Geometry: final body of the model. Coordinates: model frame, mm. A direction names the side the tool comes from. Give positions to 0.01 mm unless a question says otherwise; leave off trailing zeros. Write each loop counter-clockwise with the first axis right and the second up, starting at its lowest first coordinate (ties: lowest second). Pieces come first, ordered by that corner, then holes. Notation, with made-up numbers: (1, 64) - (21, 64) arc R26 cw to (21, 101) - close; hole circle Ø4 at (5.5, 23.5). An arc over 180 degrees is marked (long way). Return JSON: item names as keys, results as strings.
from build123d import *

# Parameters (mm, degrees)
BOSS_EXTRUDE5_DEPTH = 234.9999999
SKETCH4_W           = 42.5
SKETCH4_H           = 48.09999997
CUT_EXTRUDE1_DEPTH  = 2.000000064


with BuildPart() as part:
    # Sketch1 → Boss-Extrude5 (new body)
    with BuildSketch(Plane(origin=(0, 0, 0), x_dir=(1, 0, 0), z_dir=(0, 1, 0))):
        Polygon((-117.504462868, 326.155640462), (117.504462868, 326.155640462), (263.000000064, 160.754471715), (263.000000064, 45.003453118), (261, 45.003453118), (261, 160), (116.600094822, 324.155640398), (-116.600094822, 324.155640398), (-261, 160), (-261, 45.001214275), (-263.000000064, 45.001214275), (-263.000000064, 160.754471715), align=None)
    extrude(amount=BOSS_EXTRUDE5_DEPTH)

    # Sketch4 → Cut-Extrude1 (cut)
    with BuildSketch(Plane(origin=(0, 0, -326.155640462), x_dir=(-1, 0, 0), z_dir=(0, 0, -1))):
        with Locations((0, 87.449999931)):
            Rectangle(SKETCH4_W, SKETCH4_H)
        Polygon((-25, 63.399999946), (-25, 28.4), (25, 28.4), (25, 63.399999946), (21.25, 63.399999946), (-21.25, 63.399999946), align=None)
        Polygon((-25, 28.4), (-35, 28.4), (-35, 0), (35, 0), (35, 28.4), (25, 28.4), align=None)
    extrude(amount=-CUT_EXTRUDE1_DEPTH, mode=Mode.SUBTRACT)


solid = part.part
Q1. Mould query, pull axis X, two halves, no side actions, for faces 1 (the flat face through (-2, 116, -326.156)), 2 (the flat face through (263, 116, -104)), 3 (the flat face through (-261, 116, -103)). Classes: pulls with the +X half, pulls with the -X half, needs draft (parallel to the pull), parting line crosses it, or undercut.
Answer key:
{"face 1": "needs draft", "face 2": "pulls with the +X half", "face 3": "undercut"}
Q2. Pin query (flat end, axial travel): P1, Ø1, axis at y = 15.5, z = -325, coming from the +X side; P2, Ø1.6, axis at x = -6, z = -325.5, coming from the -Y side; P3, Ø5, axis at x = -143, y = 76, coming from the +Z side. Return the tip coordinate at first contact, or that it passes through.
Answer key:
{"P1": "stops at x = 118.96", "P2": "stops at y = 111.5", "P3": "stops at z = -291.3"}
Q3. Section query B-B, the plane z = -94. Return the cut outline in (x, y), plus the area to 3 significant figures.
Answer key:
{"outline": "(-263, 0) - (-261, 0) - (-261, 235) - (-263, 235) - close; (261, 0) - (263, 0) - (263, 235) - (261, 235) - close", "area": "940 mm^2"}
Q4. Material intervals for probe 1 along X at (y, z) = (173, -146); probe 2 along Z at (x, y) = (-42, 121.5); probe 3 along X at (y, z) = (211, -251), sorted ascending. Write a range as [from, to].
Answer key:
{"probe 1": "x = [-263, -261], [261, 263]", "probe 2": "z = [-326.16, -324.16]", "probe 3": "x = [-183.62, -180.95], [180.95, 183.62]"}
Q5. Section query D-D, the plane x = 111. Return the cut outline in (y, z), plus the area to 3 significant figures.
Answer key:
{"outline": "(0, -326.16) - (235, -326.16) - (235, -324.16) - (0, -324.16) - close", "area": "470 mm^2"}
Q6. Section query C-C, the plane y = 91.5. Return the cut outline in (x, z).
Answer key:
{"outline": "(-263, -160.75) - (-117.5, -326.16) - (-21.25, -326.16) - (-21.25, -324.16) - (-116.6, -324.16) - (-261, -160) - (-261, -45) - (-263, -45) - close; (21.25, -326.16) - (117.5, -326.16) - (263, -160.75) - (263, -45) - (261, -45) - (261, -160) - (116.6, -324.16) - (21.25, -324.16) - close"}
Q7. Section query A-A, the plane y = 36.5. Return the cut outline in (x, z), plus the area to 3 significant figures.
Answer key:
{"outline": "(-263, -160.75) - (-117.5, -326.16) - (-25, -326.16) - (-25, -324.16) - (-116.6, -324.16) - (-261, -160) - (-261, -45) - (-263, -45) - close; (25, -326.16) - (117.5, -326.16) - (263, -160.75) - (263, -45) - (261, -45) - (261, -160) - (116.6, -324.16) - (25, -324.16) - close", "area": "1,710 mm^2"}
Q8. Set-up query: faces 4 (the flat face through (189.81, 115.85, -240.93)), 5 (the flat face through (189.234, 115.855, -244.613)). Return all of +Z, -Z, +X, -X, +Y, -Y with unobstructed straight access to the full face (end or side cutting, diameter ignored); none if empty.
Answer key:
{"face 4": "+Z, +Y, -Y", "face 5": "-Z, +X, +Y, -Y"}
